```python
from build123d import *

# Parameters (mm, degrees)
F0_W      = 50.8
F0_H      = 50.8
F1_DEPTH  = 30
F2_R      = 12.7
F3_SIZE   = 5.08
F5_DEPTH  = 20
F6_R      = 5
F7_R      = 2
F8_W      = 20
F8_H      = 20
F9_DEPTH  = 15
F10_R     = 2
F11_SIZE  = 1
F13_D     = 5
F13_DEPTH = 10
F13_TIP   = 1.5021515476
F15_D     = 5
F15_DEPTH = 10
F15_TIP   = 1.5021515476


with BuildPart() as f1:
    # F0 (on Front) → F1 (new body, symmetric)
    with BuildSketch(Plane.XZ):
        Rectangle(F0_W, F0_H)
    extrude(amount=F1_DEPTH, both=True)

    # F2
    f2_edges = [f1.edges().sort_by_distance(p)[0] for p in [
        (25.4, -30, 0),
        (-25.4, -30, 0),
        (25.4, 30, 0),
        (-25.4, 30, 0),
    ]]
    fillet(f2_edges, radius=F2_R)

    # F3
    f3_edges = [f1.edges().sort_by_distance(p)[0] for p in [
        (0, -30, 25.4),
        (0, -30, -25.4),
    ]]
    chamfer(f3_edges, length=F3_SIZE)

    # F4 (on face) → F5 (join)
    with BuildSketch(Plane.XY.offset(25.4)):
        with BuildLine():
            ThreePointArc((-10, -15), (-8.5355339059, -18.5355339059), (-5, -20))
            Line((-5, -20), (5, -20))
            ThreePointArc((5, -20), (8.5355339059, -18.5355339059), (10, -15))
            Line((10, -15), (10, 15))
            ThreePointArc((10, 15), (8.5355339059, 18.5355339059), (5, 20))
            Line((5, 20), (-5, 20))
            ThreePointArc((-5, 20), (-8.5355339059, 18.5355339059), (-10, 15))
            Line((-10, 15), (-10, -15))
        make_face()
    extrude(amount=F5_DEPTH)

    # F6
    f6_edges = [f1.edges().sort_by_distance(p)[0] for p in [
        (10, 0, 45.4),
    ]]
    fillet(f6_edges, radius=F6_R)

    # F7
    f7_edges = [f1.edges().sort_by_distance(p)[0] for p in [
        (20.32, 0, 25.4),
        (25.4, 0, 20.32),
        (25.4, 0, -20.32),
        (20.32, 0, -25.4),
    ]]
    fillet(f7_edges, radius=F7_R)

    # F8 (on face) → F9 (cut)
    with BuildSketch(Plane.YZ.offset(25.4)):
        Rectangle(F8_W, F8_H)
    extrude(amount=-F9_DEPTH, mode=Mode.SUBTRACT)

    # F10
    f10_edges = [f1.edges().sort_by_distance(p)[0] for p in [
        (17.9, 10, 10),
        (17.9, -10, 10),
        (17.9, -10, -10),
        (17.9, 10, -10),
    ]]
    fillet(f10_edges, radius=F10_R)

    # F11
    f11_edges = [f1.edges().sort_by_distance(p)[0] for p in [
        (10.4, 0, 10),
        (25.4, 0, 10),
    ]]
    chamfer(f11_edges, length=F11_SIZE)

    # F13
    with Locations(Plane.XZ.offset(30)):
        with Locations((0, 0)):
            Hole(F13_D / 2, depth=F13_DEPTH)
            with Locations((0, 0, -(F13_DEPTH + F13_TIP / 2))):  # 118° drill point
                Cone(0, F13_D / 2, F13_TIP, mode=Mode.SUBTRACT)

    # F15
    with Locations(Plane.XZ.offset(30)):
        with Locations((-7.5, 12.5)):
            Hole(F15_D / 2, depth=F15_DEPTH)
            with Locations((0, 0, -(F15_DEPTH + F15_TIP / 2))):  # 118° drill point
                Cone(0, F15_D / 2, F15_TIP, mode=Mode.SUBTRACT)


solid = f1.part
```
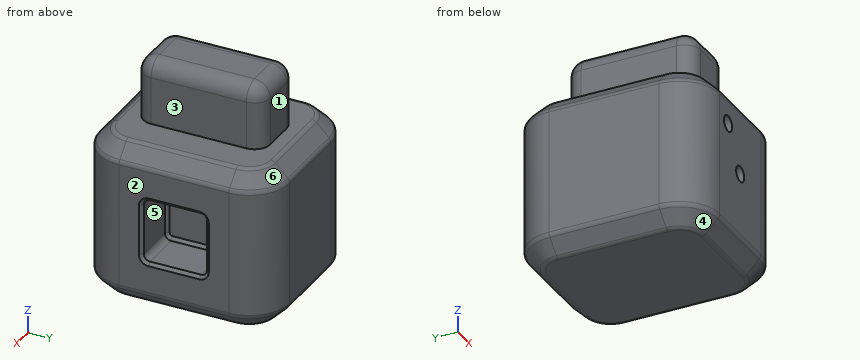
The model under review builds one solid part; all positions refer to its coordinate system, in mm. Face numbers are marked on the shaded views. A direction names the side the tool comes from. Give positions to 0.01 mm unless a question says otherwise; leave off trailing zeros. Write each loop counter-clockwise with the first axis right and the second up, starting at its lowest first coordinate (ties: lowest second). Pieces come first, ordered by that corner, then holes. Notation, with made-up numbers: (40.5, 29) - (92.5, 29) arc R29 ccw to (92.5, 59) - close; hole circle Ø9 at (15, -31.75). An arc over 180 degrees is marked (long way). Answer in a Markdown table with one row per item. Add a question column.
1. We need section A-A on z = 4.5. Write out the cut boundary in (x, y).
2. Draft analysis for pull direction Z (two halves, no side actions). For the marked faces 4, 5 and 6, state which applies: +Z half, -Z half, draft (parallel to the pull), parting line (faces both ways), or undercut.
3. Insertion check: P1, Ø5.5, axis at y = 1.5, z = 1.5, coming from the +X side; P2, Ø7.5, axis at y = 5, z = 35, coming from the +X side; P3, Ø8, axis at x = 0.5, z = 35.5, coming from the -Y side. Each pin has a flat end and moves straight along its axis. Give the tip position at first contact, or say it passes through.
4. We need section C-C on x = -4. Write out the cut boundary in (y, z), then the cut area to 3 significant figures.
5. Wall thickness on line 1 along Z through (x, y) = (17, -6.5); line 2 along Z through (x, y) = (0, -22.75); line 3 along Y through (x, z) = (13, 2.5): over which ranges is each line inside the solid? List them lowest first. Write a range as [from, to].
6. We need section B-B on x = -11.5. Write out the cut boundary in (y, z).
7. Tool access review of the marked faces 1, 2 and 3: name each direction out of +Z, -Z, +X, -X, +Y, -Y from which nothing blocks a thin tool from reaching the whole face with its end or side.
Ans:
| question | item | result |
|---|---|---|
| 1 | outline | (-25.4, -17.3) arc R12.7 ccw to (-12.7, -30) - (12.7, -30) arc R12.7 ccw to (25.4, -17.3) - (25.4, -11) - (24.4, -10) - (11.4, -10) - (10.4, -9) - (10.4, 9) - (11.4, 10) - (24.4, 10) - (25.4, 11) - (25.4, 17.3) arc R12.7 ccw to (12.7, 30) - (-12.7, 30) arc R12.7 ccw to (-25.4, 17.3) - close |
| 2 | face 4 | -Z half |
| 2 | face 5 | undercut |
| 2 | face 6 | +Z half |
| 3 | P1 | stops at x = 10.4 |
| 3 | P2 | stops at x = 10 |
| 3 | P3 | stops at y = -20 |
| 4 | outline | (-30, -19.49) arc R2 ccw to (-29.41, -20.91) - (-25.51, -24.81) arc R2 ccw to (-24.09, -25.4) - (24.09, -25.4) arc R2 ccw to (25.51, -24.81) - (29.41, -20.91) arc R2 ccw to (30, -19.49) - (30, 19.49) arc R2 ccw to (29.41, 20.91) - (25.51, 24.81) arc R2 ccw to (24.09, 25.4) - (20, 25.4) - (20, 40.4) arc R5 ccw to (15, 45.4) - (-15, 45.4) arc R5 ccw to (-20, 40.4) - (-20, 25.4) - (-24.09, 25.4) arc R2 ccw to (-25.51, 24.81) - (-29.41, 20.91) arc R2 ccw to (-30, 19.49) - close |
| 4 | area | 3,780 mm^2 |
| 5 | line 1 | z = [-25.4, -10], [10, 25.4] |
| 5 | line 2 | z = [-25.4, -2.5], [2.5, 25.4] |
| 5 | line 3 | y = [-30, -10], [10, 30] |
| 6 | outline | (-30, -19.49) arc R2 ccw to (-29.41, -20.91) - (-25.51, -24.81) arc R2 ccw to (-24.09, -25.4) - (24.09, -25.4) arc R2 ccw to (25.51, -24.81) - (29.41, -20.91) arc R2 ccw to (30, -19.49) - (30, 19.49) arc R2 ccw to (29.41, 20.91) - (25.51, 24.81) arc R2 ccw to (24.09, 25.4) - (-24.09, 25.4) arc R2 ccw to (-25.51, 24.81) - (-29.41, 20.91) arc R2 ccw to (-30, 19.49) - close |
| 7 | face 1 | +Z, +X, -X, +Y |
| 7 | face 2 | +Z, -Z, +X, +Y, -Y |
| 7 | face 3 | +Z, +X, +Y, -Y |
